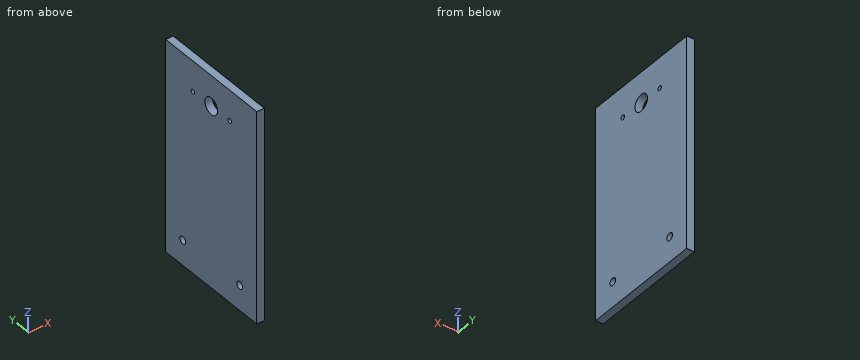
from build123d import *

# Parameters (mm, degrees)
SKETCH1_W           = 80
SKETCH1_H           = 140
SKETCH1_R           = 5.5
SKETCH1_R_2         = 1.5
SKETCH1_R_3         = 2.5
BOSS_EXTRUDE1_DEPTH = 5


with BuildPart() as part:
    # Sketch1 → Boss-Extrude1 (new body)
    with BuildSketch(Plane.YZ):
        Rectangle(SKETCH1_W, SKETCH1_H)
        with Locations((0, 49.75)):
            Circle(SKETCH1_R, mode=Mode.SUBTRACT)
        with Locations((-16.22, 49.75)):
            Circle(SKETCH1_R_2, mode=Mode.SUBTRACT)
        with Locations((16.22, 49.75)):
            Circle(SKETCH1_R_2, mode=Mode.SUBTRACT)
        with Locations((-25, -53.4)):
            Circle(SKETCH1_R_3, mode=Mode.SUBTRACT)
        with Locations((25, -53.4)):
            Circle(SKETCH1_R_3, mode=Mode.SUBTRACT)
    extrude(amount=BOSS_EXTRUDE1_DEPTH)


solid = part.part
Could you check a few things on this model? Use its own coordinates, in mm. Round coordinates to 2 decimals unless told otherwise and drop trailing zeros. Write each loop counter-clockwise with the first axis right and the second up, starting at its lowest first coordinate (ties: lowest second). Pieces come first, ordered by that corner, then holes. Notation, with made-up numbers: (34.25, 65.25) - (91.25, 65.25) arc R23 ccw to (91.25, 97.25) - close; hole circle Ø8 at (0.25, 34.25). An arc over 180 degrees is marked (long way). Use a Markdown table: item, result.
Q1. Please list where these lines run through material, in increasing order: L1, parallel to Y at x = 4.45, z = 49.5; L2, parallel to Y at x = 3.35, z = -52; L3, parallel to Z at x = 2.7, y = 16.22.
Output values:
| item | result |
|---|---|
| L1 | -40 to -17.7, -14.74 to -5.49, 5.49 to 14.74, 17.7 to 40 |
| L2 | -40 to -27.07, -22.93 to 22.93, 27.07 to 40 |
| L3 | -70 to 48.25, 51.25 to 70 |
Q2. I want a section at C-C (y = -25). List the corners of the cut face in (x, z) for me.
Output values:
| item | result |
|---|---|
| outline | (0, -70) - (5, -70) - (5, -55.9) - (0, -55.9) - close; (0, -50.9) - (5, -50.9) - (5, 70) - (0, 70) - close |
Q3. For pin 1 (5 mm diameter, centred on y = 16.22, z = 49.75, fed in from +X), with a flat end and sliding along its axis, tell me the tip position at first contact or that it passes through.
Output values:
| item | result |
|---|---|
| pin 1 | x = 5 |
Q4. I want a section at A-A (y = -16.22). List the corners of the cut face in (x, z) for me, plus the area to 3 significant figures.
Output values:
| item | result |
|---|---|
| outline | (0, -70) - (5, -70) - (5, 48.25) - (0, 48.25) - close; (0, 51.25) - (5, 51.25) - (5, 70) - (0, 70) - close |
| area | 685 mm2 |
Q5. I want a section at B-B (z = 49.75). List the corners of the cut face in (x, y) for me, plus the area to 3 significant figures.
Output values:
| item | result |
|---|---|
| outline | (0, -40) - (5, -40) - (5, -17.72) - (0, -17.72) - close; (0, -14.72) - (5, -14.72) - (5, -5.5) - (0, -5.5) - close; (0, 5.5) - (5, 5.5) - (5, 14.72) - (0, 14.72) - close; (0, 17.72) - (5, 17.72) - (5, 40) - (0, 40) - close |
| area | 315 mm2 |
